For this review, take the finished solid that the model builds, in its own axes (mm). Give positions to 0.01 mm unless a question says otherwise; leave off trailing zeros. Order: outer loops, then holes, each group sorted by start corner. A loop starts at its lowest first (then second) coordinate and runs counter-clockwise, first axis right, second up. Notation, with made-up numbers: (88.25, 86) - (142.25, 86) arc R26 cw to (142.25, 116) - close; hole circle Ø4 at (37.5, 20.25). An arc over 180 degrees is marked (long way). Use a Markdown table: item, result. Add a question column.
1) Clearance check with flat-ended pins moving along their axes: P1, Ø2.5, axis at x = 0, y = 0, coming from the +Z side; P2, Ø3, axis at x = 0, y = 0, coming from the +Z side; P3, Ø2, axis at y = -2, z = -163, coming from the +X side. State where each tip first meets the part, or that it passes through.
2) We need section A-A on z = -119. Write out the cut boundary in (x, y).
3) Wall thickness on L1, parallel to Y at x = 0, z = -8; L2, parallel to Y at x = 1.05, z = -192.5; L3, parallel to Y at x = 0.4, z = -32.5: over which ranges is each line inside the solid? List them lowest first.
```python
from build123d import *

# Parameters (mm, degrees)
SCHIZZO1_R                   = 2.5
ESTRUSIONE_ESTRUSIONE1_DEPTH = 202
FORO_PER_VITE_M3_1_D         = 3.4
FORO_PER_VITE_M3_1_DEPTH     = 9.978536948
FORO_PER_VITE_M3_1_TIP       = 1.021463052
FORO_PER_VITE_M3_2_D         = 3.4
FORO_PER_VITE_M3_2_DEPTH     = 9.978536948
FORO_PER_VITE_M3_2_TIP       = 1.021463052


with BuildPart() as part:
    # Schizzo1 → Estrusione-Estrusione1 (new body)
    with BuildSketch(Plane.XY):
        Circle(SCHIZZO1_R)
    extrude(amount=-ESTRUSIONE_ESTRUSIONE1_DEPTH)

    # Foro per Vite M3-1
    with Locations(Plane.XY):
        with Locations((0, 0)):
            Hole(FORO_PER_VITE_M3_1_D / 2, depth=FORO_PER_VITE_M3_1_DEPTH)
            with Locations((0, 0, -(FORO_PER_VITE_M3_1_DEPTH + FORO_PER_VITE_M3_1_TIP / 2))):  # 118° drill point
                Cone(0, FORO_PER_VITE_M3_1_D / 2, FORO_PER_VITE_M3_1_TIP, mode=Mode.SUBTRACT)

    # Foro per Vite M3-2
    with Locations(Plane(origin=(0, 0, -202), x_dir=(-1, 0, 0), z_dir=(0, 0, -1))):
        with Locations((0, 0)):
            Hole(FORO_PER_VITE_M3_2_D / 2, depth=FORO_PER_VITE_M3_2_DEPTH)
            with Locations((0, 0, -(FORO_PER_VITE_M3_2_DEPTH + FORO_PER_VITE_M3_2_TIP / 2))):  # 118° drill point
                Cone(0, FORO_PER_VITE_M3_2_D / 2, FORO_PER_VITE_M3_2_TIP, mode=Mode.SUBTRACT)


solid = part.part
```
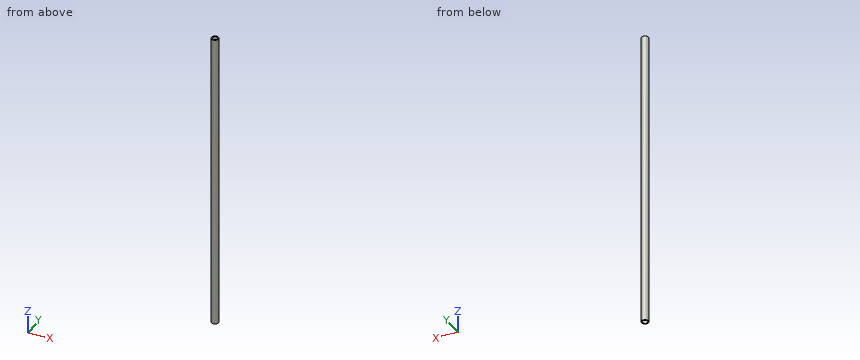
Checked values:
| question | item | result |
|---|---|---|
| 1 | P1 | z = -10.25 |
| 1 | P2 | z = -10.1 |
| 1 | P3 | x = 2.29 |
| 2 | outline | circle Ø5 at (0, 0) |
| 3 | L1 | -2.5 to -1.7, 1.7 to 2.5 |
| 3 | L2 | -2.27 to -1.34, 1.34 to 2.27 |
| 3 | L3 | -2.47 to 2.47 |
